```python
from build123d import *

# Parameters (mm, degrees)
SKETCH1_W                    = 88.9
SKETCH1_H                    = 38.1
SKETCH1_R                    = 3.556
BASE_FLANGE1_DEPTH           = 3.175
EDGE_FLANGE1_STRIP_W         = 20.82
EDGE_FLANGE1_STRIP_H         = 3.175
EDGE_FLANGE1_STRIP_CUT_DEPTH = 38.1
EDGE_FLANGE1_DEPTH           = 38.1
SKETCH9_R                    = 3.556
CUT_EXTRUDE1_DEPTH           = 147.910238326


# Sheet-metal steps are written as plain solids
with BuildPart() as part:
    # Sketch1 → Base-Flange1 (new body)
    with BuildSketch(Plane.XY):
        with Locations((-57.15, 88.9)):
            Rectangle(SKETCH1_W, SKETCH1_H)
        with Locations((-88.9, 88.9)):
            Circle(SKETCH1_R, mode=Mode.SUBTRACT)
    extrude(amount=BASE_FLANGE1_DEPTH)

    # Edge-Flange1 strip (across the edge) → Edge-Flange1 strip cut (cut)
    with BuildSketch(Plane(origin=(-12.7, 69.85, 3.175), x_dir=(-1, 0, 0), z_dir=(0, 1, 0))):
        with Locations((-3.175, -1.5875)):
            Rectangle(EDGE_FLANGE1_STRIP_W, EDGE_FLANGE1_STRIP_H)
    extrude(amount=EDGE_FLANGE1_STRIP_CUT_DEPTH, mode=Mode.SUBTRACT)

    # Edge-Flange1 section (across the edge) → Edge-Flange1 (add)
    with BuildSketch(Plane(origin=(-12.7, 69.85, 3.175), x_dir=(-1, 0, 0), z_dir=(0, 1, 0))):
        with BuildLine():
            Line((0, 4.06), (0, 47.625))
            Line((0, 47.625), (3.175, 47.625))
            Line((3.175, 47.625), (3.175, 4.06))
            ThreePointArc((3.175, 4.06), (4.364146468, 1.189146468), (7.235, 0))
            Line((7.235, 0), (7.235, -3.175))
            ThreePointArc((7.235, -3.175), (2.119082438, -1.055917562), (0, 4.06))
        make_face()
    extrude(amount=EDGE_FLANGE1_DEPTH)

    # Sketch9 → Cut-Extrude1 (cut, through all)
    with BuildSketch(Plane.ZY.offset(15.875)):
        with Locations((25.4, 88.9)):
            Circle(SKETCH9_R)
    extrude(amount=-CUT_EXTRUDE1_DEPTH, mode=Mode.SUBTRACT)


solid = part.part
```
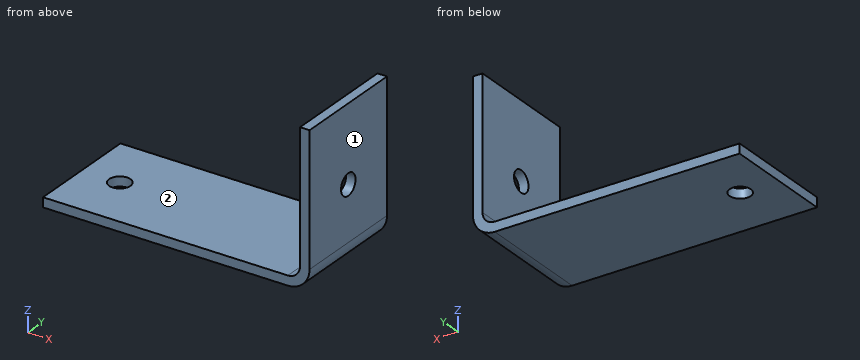
Model file for the job. Use its own axes, mm. Face numbers are marked on the shaded views. A direction names the side the tool comes from. Coordinates: 2 decimals unless noted, no trailing zeros. Loops run counter-clockwise (first coordinate to the right, second up) from the corner with the lowest first, then second, coordinate; pieces in that order, holes last. Notation, with made-up numbers: (37.5, 87.5) - (96.5, 87.5) arc R38 cw to (96.5, 126.5) - close; hole circle Ø4 at (65.25, 37.5). An arc over 180 degrees is marked (long way). Answer as a JSON object with one key per item and string values. Group by question number.
(1) Tool access for the marked faces 1 and 2: list every direction of +Z, -Z, +X, -X, +Y, -Y with a clear straight run to the whole face (end or side of a thin tool).
(2) Flat gauge pins, fed straight in: pin 1 (10 mm diameter, centred on y = 88, z = 34, fed in from -X) (3 decimals); pin 2 (19 mm diameter, centred on x = -79, y = 84, fed in from +Z) (3 decimals). Where does each tip first touch, or does it go through?
(3) Cut at D-D (y = 77.5). Give the cut face in (x, z) (3 decimals).
(4) Probe line 1 along Y through (x, z) = (-14.6, 25.4); line 2 along Z through (x, y) = (-95.5, 100) (3 decimals); line 3 along Y through (x, z) = (-88, 2). List the from-to ranges inside material, lowest first.
(5) Cut at B-B (y = 88.9). Give the cut face in (x, z) (3 decimals).
(6) Cut at A-A (z = 25.4). Give the cut face in (x, y) (3 decimals), then the cut area to 3 significant figures.
(7) Cut at C-C (x = -88.9). Give the cut face in (y, z) (3 decimals).
Geometry says:
{
 "1": {"face 1": "+Z, -Z, +X, +Y, -Y", "face 2": "+Z, -X, +Y, -Y"},
 "2": {"pin 1": "stops at x = -15.875", "pin 2": "stops at z = 3.175"},
 "3": {"outline": "(-101.6, 0) - (-19.935, 0) arc R7.235 ccw to (-12.7, 7.235) - (-12.7, 50.8) - (-15.875, 50.8) - (-15.875, 7.235) arc R4.06 cw to (-19.935, 3.175) - (-101.6, 3.175) - close"},
 "4": {"line 1": "y = 69.85 to 85.34, 92.46 to 107.95", "line 2": "z = 0 to 3.175", "line 3": "y = 69.85 to 85.46, 92.34 to 107.95"},
 "5": {"outline": "(-101.6, 0) - (-92.456, 0) - (-92.456, 3.175) - (-101.6, 3.175) - close; (-85.344, 0) - (-19.935, 0) arc R7.235 ccw to (-12.7, 7.235) - (-12.7, 21.844) - (-15.875, 21.844) - (-15.875, 7.235) arc R4.06 cw to (-19.935, 3.175) - (-85.344, 3.175) - close; (-15.875, 28.956) - (-12.7, 28.956) - (-12.7, 50.8) - (-15.875, 50.8) - close"},
 "6": {"outline": "(-15.875, 69.85) - (-12.7, 69.85) - (-12.7, 85.344) - (-15.875, 85.344) - close; (-15.875, 92.456) - (-12.7, 92.456) - (-12.7, 107.95) - (-15.875, 107.95) - close", "area": "98.4 mm^2"},
 "7": {"outline": "(69.85, 0) - (85.344, 0) - (85.344, 3.175) - (69.85, 3.175) - close; (92.456, 0) - (107.95, 0) - (107.95, 3.175) - (92.456, 3.175) - close"}
}
